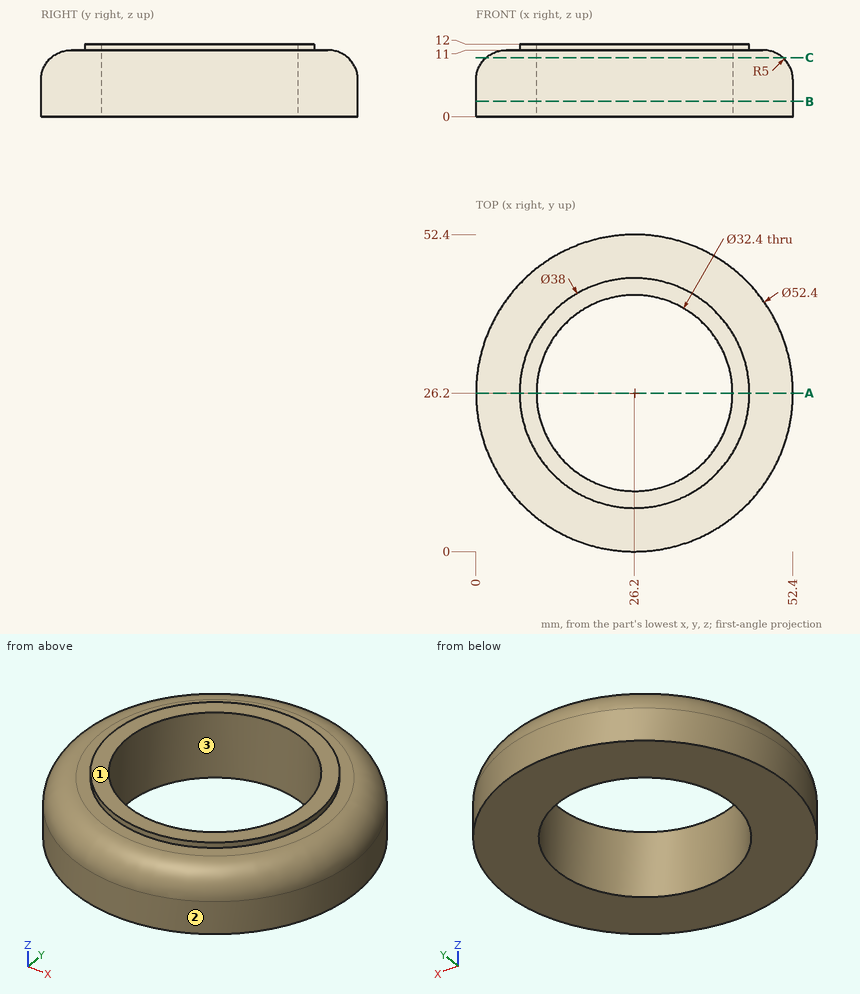
Source: three-view drawing plus pictorial views. Frame: mm from the lowest corner of the part. Round coordinates to 2 decimals unless told otherwise and drop trailing zeros. Order: outer loops, then holes, each group sorted by start corner. A loop starts at its lowest first (then second) coordinate and runs counter-clockwise, first axis right, second up. Notation, with made-up numbers: M -8,-39.75 L 37,-39.75 A34 ccw 37,-9.75 Z; hole C 28,82.25 d10. An arc over 180 degrees is marked long. One line per item, written item: value.
(1) Line query: probe 1 along Y at (x, z) = (26.2, 3.25); probe 2 along X at (y, z) = (29, 2.25); probe 3 along Y at (x, z) = (16.5, 8.5). Output: solid intervals per line, ascending. Write a range as [from, to].
Result sheet:
probe 1: [0, 10], [42.4, 52.4]
probe 2: [0.15, 10.24], [42.16, 52.25]
probe 3: [2.58, 13.23], [39.17, 49.82]
(2) Cut plane A-A (y = 26.2). Return the cut outline in (x, z).
Result sheet:
outline: M 0,0 L 10,0 L 10,12 L 7.2,12 L 7.2,11 L 5,11 A5 ccw 0,6 Z; M 42.4,0 L 52.4,0 L 52.4,6 A5 ccw 47.4,11 L 45.2,11 L 45.2,12 L 42.4,12 Z
(3) Cut plane C-C (z = 9.75). Return the cut outline in (x, y), and give its area (3 significant figures).
Result sheet:
outline: C 26.2,26.2 d49.01; hole C 26.2,26.2 d32.4
area: 1,060 mm2
(4) Cut plane B-B (z = 2.5). Return the cut outline in (x, y), and give its area (3 significant figures).
Result sheet:
outline: C 26.2,26.2 d52.4; hole C 26.2,26.2 d32.4
area: 1,330 mm2
(5) Pin query (flat end, axial travel): P1, Ø6, axis at y = 35, z = 8.5, coming from the +X side; P2, Ø5, axis at x = 23.5, z = 9, coming from the -Y side; P3, Ø3, axis at x = 25.5, z = 6, coming from the +Y side; P4, Ø12.5, axis at x = 32, y = 30, coming from the +Z side. Return the tip coordinate at first contact, or that it passes through.
Result sheet:
P1: x = 51.56
P2: y = 0.11
P3: y = 52.4
P4: through
(6) Pull-direction query (X, two-part tool) for the marked faces 1, 2 and 3; classes: pulls with the +X half, pulls with the -X half, needs draft (parallel to the pull), parting line crosses it, or undercut.
Result sheet:
face 1: needs draft
face 2: parting line crosses it
face 3: undercut
